Here's how the part is built. I have some questions about the finished solid (model axes, mm). Round coordinates to 2 decimals unless told otherwise and drop trailing zeros. Order: outer loops, then holes, each group sorted by start corner. A loop starts at its lowest first (then second) coordinate and runs counter-clockwise, first axis right, second up. Notation, with made-up numbers: M 4.5,26.25 L 32.5,26.25 A14 cw 32.5,47.25 Z; hole C -3.75,49.5 d4. An arc over 180 degrees is marked long. Write item = value, one per line. Start each with the question number.
Item 1: I want a section at A-A, the plane x = 0. List the corners of the cut face in (y, z) for me, plus the area to 3 significant figures.
Item 2: Please list where these lines run through material, in increasing order: L1, parallel to X at y = -28, z = 25.9; L2, parallel to Y at x = 27.5, z = 25.5; L3, parallel to Y at x = -10.5, z = 25.35.
Item 3: I want a section at C-C, the plane y = -7. List the corners of the cut face in (x, z) for me.
Item 4: I'm going to push a flat-ended pin straight in: P1, Ø2.5, axis at x = -19.45, y = -19.45, coming from the +Z side. Where does the tip first touch, or does it pass through?
Item 5: I want a section at D-D, the plane x = -27.5. List the corners of the cut face in (y, z) for me, plus the area to 3 significant figures.
Item 6: We'd pull the mould along Y, two halves only. Please class faces 1 (the face through (7, -24, 25)), 2 (the face through (-10.963, 30.063, 25.493)), 3 (the face through (13.17, 20.66, 25.49)): pulls with the +Y half, pulls with the -Y half, needs draft (parallel to the pull), parting line crosses it, or undercut.
```python
from build123d import *

# Parameters (mm, degrees)
CYLINDER1301_R               = 1.5
CYLINDER1301_DEPTH           = 20
CYLINDER1301_PLACEMENT_ANGLE = 45
CYLINDER1300_R               = 1.5
CYLINDER1300_DEPTH           = 20
CYLINDER1296_R               = 1.5
CYLINDER1296_DEPTH           = 20
CYLINDER1296_PLACEMENT_ANGLE = 135
CYLINDER1298_R               = 1.5
CYLINDER1298_DEPTH           = 20
CYLINDER1302_R               = 1.5
CYLINDER1302_DEPTH           = 20
CYLINDER1299_R               = 1.5
CYLINDER1299_DEPTH           = 20
CYLINDER1299_PLACEMENT_ANGLE = 225
CYLINDER1297_R               = 1.5
CYLINDER1297_DEPTH           = 20
CYLINDER1297_PLACEMENT_ANGLE = 45
CYLINDER1295_R               = 1.5
CYLINDER1295_DEPTH           = 20
CYLINDER1306_R               = 2.2
CYLINDER1306_DEPTH           = 15
CYLINDER1306_PLACEMENT_ANGLE = 22.5
TUBE054_R                    = 32
TUBE054_R_2                  = 24.5
TUBE054_DEPTH                = 1


with BuildPart() as obj1:
    # Cylinder1301 → Cylinder1301 (new body)
    with BuildSketch(Plane.XY):
        Circle(CYLINDER1301_R)
    extrude(amount=CYLINDER1301_DEPTH)


with BuildPart() as obj1_1:
    # Cylinder1301 placement: moved
    add(obj1.part.moved(Location((-19.445436, 19.445436, 10))).rotate(Axis((-19.445436, 19.445436, 10), (0, 0, 1)), CYLINDER1301_PLACEMENT_ANGLE))


with BuildPart() as obj2:
    # Cylinder1300 → Cylinder1300 (new body)
    with BuildSketch(Plane(origin=(-27.5, 0, 10), x_dir=(0, 1, 0), z_dir=(0, 0, 1))):
        Circle(CYLINDER1300_R)
    extrude(amount=CYLINDER1300_DEPTH)


with BuildPart() as obj3:
    # Cylinder1296 → Cylinder1296 (new body)
    with BuildSketch(Plane.XY):
        Circle(CYLINDER1296_R)
    extrude(amount=CYLINDER1296_DEPTH)


with BuildPart() as obj3_1:
    # Cylinder1296 placement: moved
    add(obj3.part.moved(Location((-19.445436, -19.445436, 10))).rotate(Axis((-19.445436, -19.445436, 10), (0, 0, 1)), CYLINDER1296_PLACEMENT_ANGLE))


with BuildPart() as obj4:
    # Cylinder1298 → Cylinder1298 (new body)
    with BuildSketch(Plane(origin=(0, -27.5, 10), x_dir=(-1, 0, 0), z_dir=(0, 0, 1))):
        Circle(CYLINDER1298_R)
    extrude(amount=CYLINDER1298_DEPTH)


with BuildPart() as obj5:
    # Cylinder1302 → Cylinder1302 (new body)
    with BuildSketch(Plane(origin=(27.5, 0, 10), x_dir=(0, -1, 0), z_dir=(0, 0, 1))):
        Circle(CYLINDER1302_R)
    extrude(amount=CYLINDER1302_DEPTH)


with BuildPart() as obj6:
    # Cylinder1299 → Cylinder1299 (new body)
    with BuildSketch(Plane.XY):
        Circle(CYLINDER1299_R)
    extrude(amount=CYLINDER1299_DEPTH)


with BuildPart() as obj6_1:
    # Cylinder1299 placement: moved
    add(obj6.part.moved(Location((19.445436, -19.445436, 10))).rotate(Axis((19.445436, -19.445436, 10), (0, 0, 1)), CYLINDER1299_PLACEMENT_ANGLE))


with BuildPart() as obj7:
    # Cylinder1297 → Cylinder1297 (new body)
    with BuildSketch(Plane.XY):
        Circle(CYLINDER1297_R)
    extrude(amount=CYLINDER1297_DEPTH)


with BuildPart() as obj7_1:
    # Cylinder1297 placement: moved
    add(obj7.part.moved(Location((19.445436, 19.445436, 10))).rotate(Axis((19.445436, 19.445436, 10), (0, 0, -1)), CYLINDER1297_PLACEMENT_ANGLE))


with BuildPart() as compound:
    # Cylinder1295 → Cylinder1295 (new body)
    with BuildSketch(Plane(origin=(0, 27.5, 10), x_dir=(1, 0, 0), z_dir=(0, 0, 1))):
        Circle(CYLINDER1295_R)
    extrude(amount=CYLINDER1295_DEPTH)

    # Compound: union obj1, obj2, obj3, obj4, obj5, obj6, obj7
    add(obj1_1.part)
    add(obj2.part)
    add(obj3_1.part)
    add(obj4.part)
    add(obj5.part)
    add(obj6_1.part)
    add(obj7_1.part)


with BuildPart() as obj8:
    # Cylinder1306 → Cylinder1306 (new body)
    with BuildSketch(Plane.XY):
        Circle(CYLINDER1306_R)
    extrude(amount=CYLINDER1306_DEPTH)


with BuildPart() as obj8_1:
    # Cylinder1306 placement: moved
    add(obj8.part.moved(Location((12.24587, -29.564145, 20))).rotate(Axis((12.24587, -29.564145, 20), (0, 0, 1)), CYLINDER1306_PLACEMENT_ANGLE))


with BuildPart() as cut492:
    # Tube054 → Tube054 (new body)
    with BuildSketch(Plane.XY.offset(25)):
        Circle(TUBE054_R)
        Circle(TUBE054_R_2, mode=Mode.SUBTRACT)
    extrude(amount=TUBE054_DEPTH)

    # Cut497: cut obj8
    add(obj8_1.part, mode=Mode.SUBTRACT)

    # Cut492: cut Compound
    add(compound.part, mode=Mode.SUBTRACT)


solid = cut492.part
```
Filled in:
q1.outline = M -32,25 L -29,25 L -29,26 L -32,26 Z; M -26,25 L -24.5,25 L -24.5,26 L -26,26 Z; M 24.5,25 L 26,25 L 26,26 L 24.5,26 Z; M 29,25 L 32,25 L 32,26 L 29,26 Z
q1.area = 9.00 mm^2
q2.L1 = -15.49 to -1.41, 1.41 to 10.7, 13.79 to 15.49
q2.L2 = -16.36 to -1.5, 1.5 to 16.36
q2.L3 = -30.23 to -22.14, 22.14 to 30.23
q3.outline = M -31.22,25 L -23.48,25 L -23.48,26 L -31.22,26 Z; M 23.48,25 L 31.22,25 L 31.22,26 L 23.48,26 Z
q4.P1 = through
q5.outline = M -16.36,25 L -1.5,25 L -1.5,26 L -16.36,26 Z; M 1.5,25 L 16.36,25 L 16.36,26 L 1.5,26 Z
q5.area = 29.7 mm^2
q6.face_1 = needs draft
q6.face_2 = parting line crosses it
q6.face_3 = undercut
